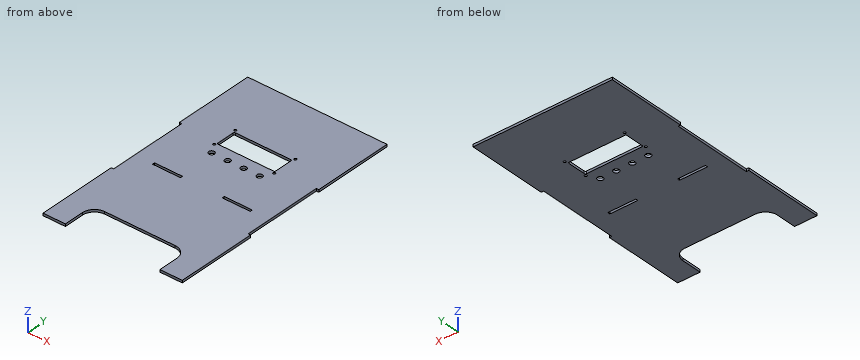
Autodesk Inventor part; units mm, degrees
ref_plane "YZ Plane" through (0, 0, 0) normal (1, 0, 0) x (0, 1, 0)
ref_plane "XZ Plane" through (0, 0, 0) normal (0, 1, 0) x (-1, 0, 0)
ref_plane "XY Plane" through (0, 0, 0) normal (0, 0, 1) x (1, 0, 0)
sketch "Sketch1" plane through (0, 0, 0) normal (0, 0, 1) x (1, 0, 0)
  line L0 (-84, -131.5) -> (84, -131.5)
  line L1 (84, -131.5) -> (84, 168.5)
  line L2 (84, 168.5) -> (-84, 168.5)
  line L3 (-84, 168.5) -> (-84, -131.5)
  line L4 (-84, 1.5) -> (-84, -1.5)
  line L5 (84, -1.5) -> (84, 1.5)
  line L6 (61, -1.5) -> (84, -1.5)
  line L7 (26, -1.5) -> (61, -1.5)
  line L8 (61, 1.5) -> (61, -1.5)
  line L9 (26, 1.5) -> (61, 1.5)
  line L10 (26, 1.5) -> (26, -1.5)
  point P0 (0, 0)
  dimension "d0" = 300
  dimension "d1" = 170
extrude "Extrusion1" add sketch "Sketch1" along normal blind 3
sketch "Sketch2" plane through (0, 0, 0) normal (0, 0, -1) x (-1, 0, 0)
  line L0 (84, 1.5) -> (84, -1.5)
  line L1 (84, -1.5) -> (61, -1.5)
  line L2 (61, 1.5) -> (61, -1.5)
  line L3 (26, 1.5) -> (61, 1.5)
  line L4 (26, -1.5) -> (26, 1.5)
  line L5 (26, -1.5) -> (-26, -1.5)
  line L6 (-26, 1.5) -> (-26, -1.5)
  line L7 (-61, 1.5) -> (-26, 1.5)
  line L8 (-61, -1.5) -> (-61, 1.5)
  line L9 (-61, -1.5) -> (-84, -1.5)
  line L10 (-84, -1.5) -> (-84, 1.5)
  line L11 (-84, 1.5) -> (-61, 1.5)
  line L12 (61, 1.5) -> (84, 1.5)
  line L13 (61, -1.5) -> (26, -1.5)
  line L14 (-26, 1.5) -> (26, 1.5)
  line L15 (-26, -1.5) -> (-61, -1.5)
  point P0 (0, 0)
extrude "Extrusion2" cut sketch "Sketch2" against normal blind 10 contours L2 L13 L4 L3
sketch "Sketch3" plane through (0, 0, 3) normal (0, 0, 1) x (1, 0, 0)
  line L0 (84, -131.5) -> (84, 168.5)
  line L1 (84, -131.5) -> (87, -131.5)
  line L2 (87, -131.5) -> (87, -31.5)
  line L3 (87, -31.5) -> (84, -31.5)
  line L4 (84, -31.5) -> (84, -131.5)
  line L5 (-61, -1.5) -> (-26, -1.5)
  line L6 (-26, -1.5) -> (-26, 1.5)
  line L7 (-26, 1.5) -> (-61, 1.5)
  line L8 (-61, 1.5) -> (-61, -1.5)
  line L9 (26, 1.5) -> (26, -1.5)
  line L10 (26, -1.5) -> (61, -1.5)
  line L11 (61, -1.5) -> (61, 1.5)
  line L12 (61, 1.5) -> (26, 1.5)
  line L13 (-84, 168.5) -> (84, 168.5)
  line L14 (84, 168.5) -> (84, -131.5)
  line L15 (84, -131.5) -> (-84, -131.5)
  line L16 (-84, -131.5) -> (-84, 168.5)
  line L17 (87, 168.5) -> (84, 168.5)
  line L18 (84, 68.5) -> (87, 68.5)
  line L19 (87, 68.5) -> (87, 168.5)
  line L20 (84, 168.5) -> (84, 68.5)
  line L21 (-84, -31.5) -> (-87, -31.5)
  line L22 (-87, -131.5) -> (-84, -131.5)
  line L23 (-84, -131.5) -> (-84, -31.5)
  line L24 (-87, -31.5) -> (-87, -131.5)
  line L25 (-84, 168.5) -> (-87, 168.5)
  line L26 (-87, 68.5) -> (-84, 68.5)
  line L27 (-84, 68.5) -> (-84, 168.5)
  line L28 (-87, 168.5) -> (-87, 68.5)
  point P0 (0, 0)
  dimension "d6" = 100
  dimension "d7" = 3
  dimension "d10" = 200
  dimension "d13" = 171
extrude "Extrusion3" add sketch "Sketch3" against normal up to surface (3 mm away) contours L0 L3 L2 L1 | L22 L24 L21 L16 | L0 L17 L19 L18 | L26 L28 L25 L16
sketch "Sketch4" plane through (0, 0, 3) normal (0, 0, 1) x (1, 0, 0)
  line L0 (-59, -131.5) -> (59, -131.5)
  line L1 (59, -131.5) -> (59, -91.5)
  line L2 (59, -91.5) -> (-59, -91.5)
  line L3 (-59, -91.5) -> (-59, -131.5)
  line L4 (-87, -131.5) -> (87, -131.5)
  line L5 (87, -131.5) -> (87, -31.5)
  line L6 (-87, -31.5) -> (-87, -131.5)
  point P0 (0, 0)
  dimension "d18" = 28
  dimension "d19" = 28
  dimension "d20" = 40
extrude "Extrusion4" cut sketch "Sketch4" against normal blind 10
fillet "Fillet1" radius 15 2 edges at (59, -91.5, 1.5) (-59, -91.5, 1.5)
sketch "Sketch5" plane through (0, 0, 0) normal (0, 0, -1) x (-1, 0, 0)
  circle A0 centre (-29.3933, 49.5) radius 3.5
  circle A1 centre (-9.3933, 49.5) radius 3.5
  circle A2 centre (10.6067, 49.5) radius 3.5
  circle A3 centre (30.6067, 49.5) radius 3.5
  line L0 (-34.0433, 89.15) -> (35.2567, 89.15)
  arc A4 (36.2567, 88.15) -> (35.2567, 89.15) centre (35.2567, 88.15) ccw
  line L1 (36.2567, 88.15) -> (36.2567, 65.85)
  arc A5 (35.2567, 64.85) -> (36.2567, 65.85) centre (35.2567, 65.85) ccw
  line L2 (35.2567, 64.85) -> (-34.0433, 64.85)
  arc A6 (-35.0433, 65.85) -> (-34.0433, 64.85) centre (-34.0433, 65.85) ccw
  line L3 (-35.0433, 65.85) -> (-35.0433, 88.15)
  arc A7 (-34.0433, 89.15) -> (-35.0433, 88.15) centre (-34.0433, 88.15) ccw
  line L4 (-34.5433, 88.15) -> (-34.5433, 65.85)
  arc A8 (-34.5433, 65.85) -> (-34.0433, 65.35) centre (-34.0433, 65.85) ccw
  line L5 (-34.0433, 65.35) -> (35.2567, 65.35)
  arc A9 (35.2567, 65.35) -> (35.7567, 65.85) centre (35.2567, 65.85) ccw
  line L6 (35.7567, 65.85) -> (35.7567, 88.15)
  arc A10 (35.7567, 88.15) -> (35.2567, 88.65) centre (35.2567, 88.15) ccw
  line L7 (35.2567, 88.65) -> (33.3925, 88.65)
  spline S0 degree 3 poles (33.3925, 88.65) (33.3126, 88.65) (33.217, 88.642) (32.9717, 88.6132) (32.7737, 88.5819) (32.6067, 88.5819) knots 0.255439 0.255439 0.255439 0.255439 0.279421 0.279421 0.329528 0.329528 0.329528 0.329528
  line L8 (32.6067, 88.5819) -> (-31.3933, 88.5819)
  spline S1 degree 3 poles (-31.3933, 88.5819) (-31.5603, 88.5819) (-31.7583, 88.6132) (-32.0036, 88.642) (-32.0992, 88.65) (-32.1791, 88.65) knots 0.329528 0.329528 0.329528 0.329528 0.379635 0.379635 0.403617 0.403617 0.403617 0.403617
  line L9 (-32.1791, 88.65) -> (-34.0433, 88.65)
  arc A11 (-34.0433, 88.65) -> (-34.5433, 88.15) centre (-34.0433, 88.15) ccw
  line L10 (-33.3933, 69) -> (-33.3933, 86)
  line L11 (-33.3933, 86) -> (34.6067, 86)
  line L12 (34.6067, 86) -> (34.6067, 69)
  line L13 (34.6067, 69) -> (-33.3933, 69)
  circle A12 centre (38.1067, 93) radius 1.5
  circle A13 centre (-36.8933, 93) radius 1.5
  circle A14 centre (-36.8933, 62) radius 1.5
  circle A15 centre (38.1067, 62) radius 1.5
  line L14 (36.7567, 65.85) -> (36.7567, 88.15)
  arc A16 (36.7567, 88.15) -> (35.2567, 89.65) centre (35.2567, 88.15) ccw
  line L15 (35.2567, 89.65) -> (-34.0433, 89.65)
  arc A17 (-34.0433, 89.65) -> (-35.5433, 88.15) centre (-34.0433, 88.15) ccw
  line L16 (-35.5433, 88.15) -> (-35.5433, 65.85)
  arc A18 (-35.5433, 65.85) -> (-34.0433, 64.35) centre (-34.0433, 65.85) ccw
  line L17 (-34.0433, 64.35) -> (35.2567, 64.35)
  arc A19 (35.2567, 64.35) -> (36.7567, 65.85) centre (35.2567, 65.85) ccw
  point P0 (0, 0)
  dimension "d24" = 0.5
extrude "Extrusion5" cut sketch "Sketch5" against normal blind 10 contours A0 | A1 | A2 | A3 | L0 A4 L1 A5 L2 A6 L3 A7 | A11 L9 S1 L8 S0 L7 A10 L6 A9 L5 A8 L4 | L10 L11 L12 L13 | A12 | A13 | A14 | A15 | A19 L17 A18 L16 A17 L15 A16 L14
properties part number "Pared_Lateral_ConCircuito"
The listing builds one solid part. Answer for the finished solid, in the listing's coordinates (mm). Coordinates: 2 decimals unless noted, no trailing zeros. Write each loop counter-clockwise with the first axis right and the second up, starting at its lowest first coordinate (ties: lowest second). Pieces come first, ordered by that corner, then holes. Notation, with made-up numbers: (-34.75, 12) - (-15.75, 12) arc R27 cw to (-15.75, 37) - close; hole circle Ø7 at (-2.75, 35.25). An arc over 180 degrees is marked (long way). Return JSON: item names as keys, results as strings. Group by question number.
1. A cutting plane is placed at A-A, the plane y = 49.5. Determine the outline of the cut face in (x, z).
2. A cutting plane is placed at C-C, the plane x = 54. Determine the outline of the cut face in (y, z), plus the area to 3 significant figures.
3. Given pin 1 (0.9 mm diameter, centred on x = -8, z = 2, fed in from -Y); pin 2 (1.5 mm diameter, centred on y = 26.5, z = 1.5, fed in from -X); pin 3 (10 mm diameter, centred on x = -16, y = 56, fed in from -Z); pin 4 (5.5 mm diameter, centred on x = -30.61, y = 49.5, fed in from +Z), each flat-ended and moving along its own axis, determine where each tip first touches the part or whether it passes through.
4. A cutting plane is placed at B-B, the plane y = -110. Determine the outline of the cut face in (x, z).
5. A cutting plane is placed at D-D, the plane z = 1.05. Give the number of separate pieces and of enclosed holes in the cut face, plus the area to 3 significant figures.
6. Straight lines are drawn through the part: L1, parallel to Y at x = 30, z = 2.4; L2, parallel to X at y = 93, z = 1.05; L3, parallel to X at y = -114.5, z = 2.15. For each, find the intervals that lie inside material, in ascending order.
Ans:
{
 "1": {"outline": "(-84, 0) - (-34.11, 0) - (-34.11, 3) - (-84, 3) - close; (-27.11, 0) - (-14.11, 0) - (-14.11, 3) - (-27.11, 3) - close; (-7.11, 0) - (5.89, 0) - (5.89, 3) - (-7.11, 3) - close; (12.89, 0) - (25.89, 0) - (25.89, 3) - (12.89, 3) - close; (32.89, 0) - (84, 0) - (84, 3) - (32.89, 3) - close"},
 "2": {"outline": "(-95.32, 0) - (-1.5, 0) - (-1.5, 3) - (-95.32, 3) - close; (1.5, 0) - (168.5, 0) - (168.5, 3) - (1.5, 3) - close", "area": "782 mm²"},
 "3": {"pin 1": "y = -91.5", "pin 2": "x = -84", "pin 3": "z = 0", "pin 4": "through"},
 "4": {"outline": "(-87, 0) - (-59, 0) - (-59, 3) - (-87, 3) - close; (59, 0) - (87, 0) - (87, 3) - (59, 3) - close"},
 "5": {"separate pieces": "1", "enclosed holes": "11", "area": "44,800 mm²"},
 "6": {"L1": "-91.5 to -1.5, 1.5 to 46.05, 52.95 to 64.35, 89.65 to 168.5", "L2": "-87 to -39.61, -36.61 to 35.39, 38.39 to 87", "L3": "-87 to -59, 59 to 87"}
}
